Design review of the part built by this model. Coordinates are the model's own, in mm. A direction names the side the tool comes from. Round coordinates to 2 decimals unless told otherwise and drop trailing zeros. Loops run counter-clockwise (first coordinate to the right, second up) from the corner with the lowest first, then second, coordinate; pieces in that order, holes last. Notation, with made-up numbers: (-29.5, -32) - (22.5, -32) arc R26 ccw to (22.5, -15) - close; hole circle Ø8 at (60, 29). An arc over 180 degrees is marked (long way). Answer as CSV lines item,"result". Start each with the question number.
(1) Consider section C-C (y = -4.25). Give the boundary of the cut face in (x, z), and give its area (3 significant figures).
(2) Consider section A-A (x = 0). Give the boundary of the cut face in (y, z), and give its area (3 significant figures).
(3) For P1, Ø8, axis at x = 0, y = 1.5, coming from the -Z side; P2, Ø2, axis at x = -11, z = -1, coming from the -Y side, all flat-tipped, find the tip position at first contact; note any pin that passes through.
(4) For faces 4 (the flat face through (0, -4, 3.9)), 5 (the cylindrical face through (18.5, -10.07, -5.13)), list the 3-axis set-ups (+Z, -Z, +X, -X, +Y, -Y) from which the entire face can be reached by the end or side of a thin tool; tool diameter is ignored.
(5) Wall thickness on L1, parallel to Z at x = 5.5, y = -8.25; L2, parallel to X at y = 1.5, z = 5.3; L3, parallel to Y at x = -18, z = 0.25: over which ranges is each line inside the solid? List them lowest first.
(6) Consider section D-D (x = 4). Give the boundary of the cut face in (y, z).
(7) Consider section B-B (y = 1.5). Give the boundary of the cut face in (x, z), and give its area (3 significant figures).
(8) Mouldability with a two-part tool opening along Y and no side actions: class faces 1 (the cylindrical face through (18.57, -10, 5.17)), 2 (the cylindrical face through (-3, 1.6, -5.1)), 3 (the flat face through (0, -3, -6.4)) as released by +Y, released by -Y, zero draft, split by the parting line, or undercut.
from build123d import *

# Parameters (mm, degrees)
BOSS_EXTRUDE1_DEPTH            = 6.4
BOSS_EXTRUDE1_DEPTH_BACK       = 6.4
SKETCH1_W                      = 40
SKETCH1_H                      = 23
CUT_EXTRUDE1_REACH             = 25.942
SKETCH2_W                      = 7.8
SKETCH2_H                      = 20.5
CUT_EXTRUDE1_DIRECTION_2_REACH = 25.942
FILLET1_R                      = 5
FILLET2_R                      = 2.5
CUT_EXTRUDE2_REACH             = 25.942
SKETCH3_R                      = 3
CUT_EXTRUDE2_DIRECTION_2_REACH = 25.942


with BuildPart() as part:
    # Sketch1 → Boss-Extrude1 (new, two sides: drawn at the far end of the back side and taken through both)
    with BuildSketch(Plane.XY.offset(-BOSS_EXTRUDE1_DEPTH_BACK)):
        Rectangle(SKETCH1_W, SKETCH1_H)
    extrude(amount=BOSS_EXTRUDE1_DEPTH + BOSS_EXTRUDE1_DEPTH_BACK)

    # Cut-Extrude1: up to this face of the body (flat: up to its plane)
    cut_extrude1_end = Plane(part.part.faces().sort_by_distance((-20, 0, 0))[0])
    # Sketch2 → Cut-Extrude1 (cut, up to the picked face)
    with BuildSketch(Plane(origin=(0, 0, 0), x_dir=(0, 0, -1), z_dir=(1, 0, 0)), mode=Mode.PRIVATE) as cut_extrude1_sk1:
        with Locations((0, -1.25)):
            Rectangle(SKETCH2_W, SKETCH2_H)
    cut_extrude1_tool1 = split(extrude(cut_extrude1_sk1.sketch, amount=-CUT_EXTRUDE1_REACH, mode=Mode.PRIVATE), bisect_by=cut_extrude1_end, keep=Keep.BOTH, mode=Mode.PRIVATE)
    add(cut_extrude1_tool1.solids().sort_by(Axis((0, -1.25, 0), (-1, 0, 0)))[0], mode=Mode.SUBTRACT)

    # Cut-Extrude1 direction 2: up to this face of the body (flat: up to its plane)
    cut_extrude1_direction_2_end = Plane(part.part.faces().sort_by_distance((20, 0, 0))[0])
    # Sketch2 → Cut-Extrude1 direction 2 (cut, up to the picked face)
    with BuildSketch(Plane(origin=(0, 0, 0), x_dir=(0, 0, -1), z_dir=(1, 0, 0)), mode=Mode.PRIVATE) as cut_extrude1_direction_2_sk1:
        with Locations((0, -1.25)):
            Rectangle(SKETCH2_W, SKETCH2_H)
    cut_extrude1_direction_2_tool1 = split(extrude(cut_extrude1_direction_2_sk1.sketch, amount=CUT_EXTRUDE1_DIRECTION_2_REACH, mode=Mode.PRIVATE), bisect_by=cut_extrude1_direction_2_end, keep=Keep.BOTH, mode=Mode.PRIVATE)
    add(cut_extrude1_direction_2_tool1.solids().sort_by(Axis((0, -1.25, 0), (1, 0, 0)))[0], mode=Mode.SUBTRACT)

    # Fillet1
    fillet1_edges = [part.edges().sort_by_distance(p)[0] for p in [
        (-20, -11.5, 5.15),
        (20, -11.5, 5.15),
        (20, -11.5, -5.15),
        (-20, -11.5, -5.15),
    ]]
    fillet(fillet1_edges, radius=FILLET1_R)

    # Fillet2
    fillet2_edges = [part.edges().sort_by_distance(p)[0] for p in [
        (0, 11.5, 6.4),
        (0, 11.5, -6.4),
    ]]
    fillet(fillet2_edges, radius=FILLET2_R)

    # Cut-Extrude2: up to this face of the body (flat: up to its plane)
    cut_extrude2_end = Plane(part.part.faces().sort_by_distance((0, -1.128903629, -6.4))[0])
    # Sketch3 → Cut-Extrude2 (cut, up to the picked face)
    with BuildSketch(Plane.XY, mode=Mode.PRIVATE) as cut_extrude2_sk1:
        with Locations((0, 1.5)):
            Circle(SKETCH3_R)
    cut_extrude2_tool1 = split(extrude(cut_extrude2_sk1.sketch, amount=-CUT_EXTRUDE2_REACH, mode=Mode.PRIVATE), bisect_by=cut_extrude2_end, keep=Keep.BOTH, mode=Mode.PRIVATE)
    add(cut_extrude2_tool1.solids().sort_by(Axis((0, 1.5, 0), (0, 0, -1)))[0], mode=Mode.SUBTRACT)

    # Cut-Extrude2 direction 2: up to this face of the body (flat: up to its plane)
    cut_extrude2_direction_2_end = Plane(part.part.faces().sort_by_distance((0, -1.128903629, 6.4))[0])
    # Sketch3 → Cut-Extrude2 direction 2 (cut, up to the picked face)
    with BuildSketch(Plane.XY, mode=Mode.PRIVATE) as cut_extrude2_direction_2_sk1:
        with Locations((0, 1.5)):
            Circle(SKETCH3_R)
    cut_extrude2_direction_2_tool1 = split(extrude(cut_extrude2_direction_2_sk1.sketch, amount=CUT_EXTRUDE2_DIRECTION_2_REACH, mode=Mode.PRIVATE), bisect_by=cut_extrude2_direction_2_end, keep=Keep.BOTH, mode=Mode.PRIVATE)
    add(cut_extrude2_direction_2_tool1.solids().sort_by(Axis((0, 1.5, 0), (0, 0, 1)))[0], mode=Mode.SUBTRACT)


solid = part.part
Determined:
1,outline,"(-20, -6.4) - (20, -6.4) - (20, -3.9) - (-20, -3.9) - close; (-20, 3.9) - (20, 3.9) - (20, 6.4) - (-20, 6.4) - close"
1,area,"200 mm^2"
2,outline,"(-11.5, -6.4) - (-1.5, -6.4) - (-1.5, -3.9) - (-11.5, -3.9) - close; (-11.5, 3.9) - (-1.5, 3.9) - (-1.5, 6.4) - (-11.5, 6.4) - close; (4.5, -6.4) - (9, -6.4) arc R2.5 ccw to (11.5, -3.9) - (11.5, 3.9) arc R2.5 ccw to (9, 6.4) - (4.5, 6.4) - (4.5, 3.9) - (9, 3.9) - (9, -3.9) - (4.5, -3.9) - close"
2,area,"102 mm^2"
3,P1,"stops at z = -6.4"
3,P2,"stops at y = 9"
4,face 4,"+X, -X, -Y"
4,face 5,"+Z, -Z, +X, -Y"
5,L1,"z = -6.4 to -3.9, 3.9 to 6.4"
5,L2,"x = -20 to -3, 3 to 20"
5,L3,"y = 9 to 11.5"
6,outline,"(-11.5, -6.4) - (9, -6.4) arc R2.5 ccw to (11.5, -3.9) - (11.5, 3.9) arc R2.5 ccw to (9, 6.4) - (-11.5, 6.4) - (-11.5, 3.9) - (9, 3.9) - (9, -3.9) - (-11.5, -3.9) - close"
7,outline,"(-20, -6.4) - (-3, -6.4) - (-3, -3.9) - (-20, -3.9) - close; (-20, 3.9) - (-3, 3.9) - (-3, 6.4) - (-20, 6.4) - close; (3, -6.4) - (20, -6.4) - (20, -3.9) - (3, -3.9) - close; (3, 3.9) - (20, 3.9) - (20, 6.4) - (3, 6.4) - close"
7,area,"170 mm^2"
8,face 1,"released by -Y"
8,face 2,"undercut"
8,face 3,"zero draft"
